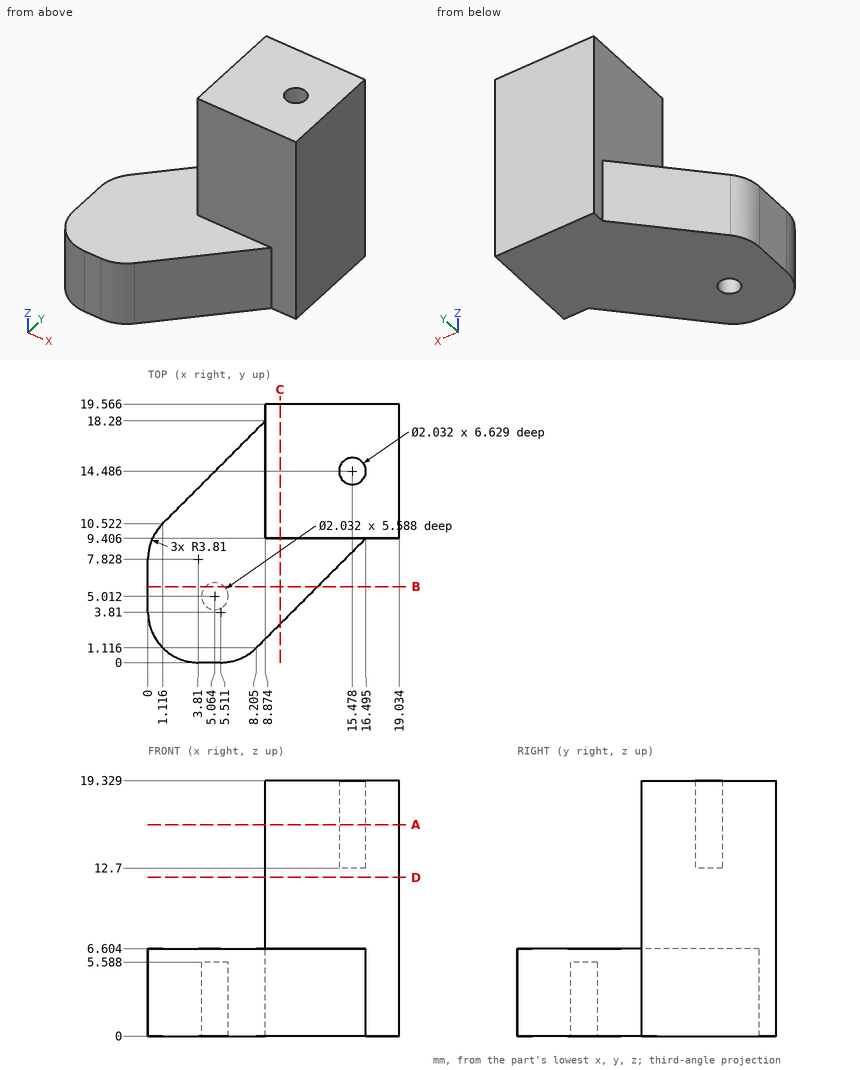
Check sheet for the drawn part. Datum: minimum x, y, z corner. Units: mm. Give positions to 0.01 mm unless a question says otherwise; leave off trailing zeros. Loops run counter-clockwise (first coordinate to the right, second up) from the corner with the lowest first, then second, coordinate; pieces in that order, holes last. Notation, with made-up numbers: M 11.25,88 L 18.25,88 A26 ccw 18.25,108 Z; hole C -34.5,73.25 d3. An arc over 180 degrees is marked long. Answer as CSV lines item,"result".
Item 1: Depth check by flat-ended pin: pin 1 Ø1 at (x, z) = (14.5, 10) entering from -Y; pin 2 Ø1.6 at (x, y) = (5.06, 5.01) entering from -Z; pin 3 Ø8 at (y, z) = (12, 9.5) entering from -X; pin 4 Ø1.5 at (x, z) = (8.5, 7) entering from +Y. Enter the tip coordinate at first touch or a pass-through.
Reply:
pin 1,"y = 9.41"
pin 2,"z = 5.59"
pin 3,"x = 0.27"
pin 4,"y = 19.57"
Item 2: Sectioned sample at C-C, the plane x = 10. Enter the section's corners in (y, z).
Reply:
outline,"M 2.91,0 L 19.57,0 L 19.57,19.33 L 9.41,19.33 L 9.41,6.6 L 2.91,6.6 Z"
Item 3: Sectioned sample at D-D, the plane z = 12. Enter the section's corners in (x, y) (1 decimal), then the cut area to 3 significant figures.
Reply:
outline,"M 8.9,9.4 L 19,9.4 L 19,19.6 L 8.9,19.6 Z"
area,"103 mm^2"
Item 4: Sectioned sample at A-A, the plane z = 16. Enter the section's corners in (x, y) (1 decimal).
Reply:
outline,"M 8.9,9.4 L 19,9.4 L 19,19.6 L 8.9,19.6 Z; hole C 15.5,14.5 d2"
Item 5: Sectioned sample at B-B, the plane y = 5.75. Enter the section's corners in (x, z).
Reply:
outline,"M 0,0 L 4.37,0 L 4.37,5.59 L 5.76,5.59 L 5.76,0 L 12.84,0 L 12.84,6.6 L 0,6.6 Z"
Item 6: Scan lines: L1, parallel to X at y = 15, z = 1 (1 decimal); L2, parallel to Y at x = 12.5, z = 9.5; L3, parallel to Z at x = 5.5, y = 13. Record each from-to range of solid material in increasing order.
Reply:
L1,"5.6 to 19"
L2,"9.41 to 19.57"
L3,"0 to 6.6"
